from build123d import *

# Parameters (mm, degrees)
F1_DEPTH = 50
F2_DEPTH = 25
F0_W     = 36
F0_H     = 20
F3_DEPTH = 10
F4_DEPTH = 10


with BuildPart() as f1:
    # F0 (on Front) → F1 (new body, symmetric)
    with BuildSketch(Plane.XZ):
        Polygon((-60, -30), (60, -30), (60, 30), (18, 30), (18, 10), (-18, 10), (-18, 30), (-60, 30), align=None)
    extrude(amount=F1_DEPTH, both=True)

    # F0 (on Front) → F2 (join, symmetric)
    with BuildSketch(Plane.XZ):
        with BuildLine():
            add(Edge.make_bspline(
                [(-60, 30), (-60, 40.4474846921), (-37.2177352662, 50), (-18, 50)],
                knots=[0, 0, 0, 0, 46.5188133985, 46.5188133985, 46.5188133985, 46.5188133985], degree=3))
            Line((-60, 30), (-18, 30))
            Line((-18, 30), (-18, 50))
        make_face()
    extrude(amount=F2_DEPTH, both=True)

    # F0 (on Front) → F3 (join, symmetric)
    with BuildSketch(Plane.XZ):
        with Locations((0, 20)):
            Rectangle(F0_W, F0_H)
    extrude(amount=F3_DEPTH, both=True)

    # F0 (on Front) → F4 (join, symmetric)
    with BuildSketch(Plane.XZ):
        with Locations((0, 40)):
            Rectangle(F0_W, F0_H)
        with BuildLine():
            Line((18, 30), (60, 30))
            Line((60, 30), (60, 56.5))
            ThreePointArc((60, 56.5), (63.954058454, 66.045941546), (73.5, 70))
            Line((73.5, 70), (87.8666490715, 70))
            Line((87.8666490715, 70), (87.8666490715, 75))
            add(Edge.make_bspline(
                [(18, 50), (18.3067479085, 75.1533858136), (72.5292141174, 78.3742428055), (87.8666490715, 75)],
                knots=[0, 0, 0, 0, 74.2047751326, 74.2047751326, 74.2047751326, 74.2047751326], degree=3))
            Line((18, 50), (18, 30))
        make_face()
    extrude(amount=F4_DEPTH, both=True)

    # F0 (on Front) → F5 (revolve)
    with BuildSketch(Plane.XZ):
        Polygon((97.8666490715, 75), (87.8666490715, 75), (87.8666490715, 70), (92.8666490715, 70), (92.8666490715, 65), (97.8666490715, 65), align=None)
    revolve(axis=Axis((87.8666490715, 0, 70), (0, 0, 1)))


solid = f1.part
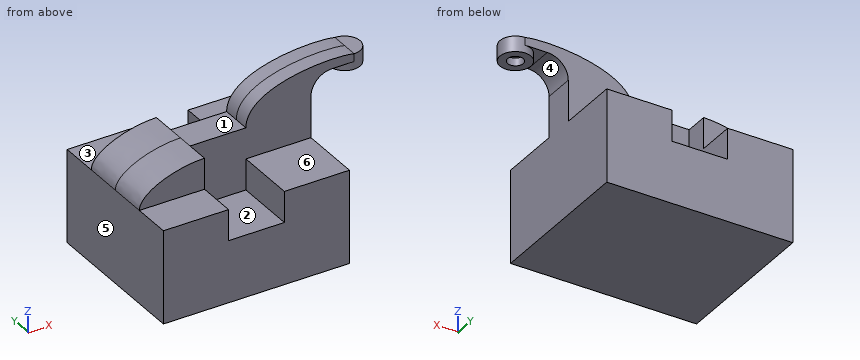
Input: part model. Units: mm. Frame: model coordinates. Face numbers are marked on the shaded views. A direction names the side the tool comes from. Coordinates: 2 decimals unless noted, no trailing zeros. Loops run counter-clockwise (first coordinate to the right, second up) from the corner with the lowest first, then second, coordinate; pieces in that order, holes last. Notation, with made-up numbers: (6, 23.5) -> (59, 23.5) arc R24 cw to (59, 62.5) -> close; hole circle Ø5 at (34, 2). An arc over 180 degrees is marked (long way). Write item = value, one per line. Start each with the question number.
Item 1: Reachability of the marked faces 1, 2 and 3 from +Z, -Z, +X, -X, +Y, -Y: full face, straight path, thin tool, end or side. Return the list, or none.
Item 2: Mould query, pull axis X, two halves, no side actions, for the marked faces 4, 5 and 6. Classes: pulls with the +X half, pulls with the -X half, needs draft (parallel to the pull), parting line crosses it, or undercut.
Item 3: Cut plane A-A, the plane z = 21. Return loops of the section in (x, y), plus the area to 3 significant figures.
Item 4: First-contact query: P1, Ø13, axis at x = 87.87, y = 0, coming from the +Z side; P2, Ø5, axis at y = 2, z = 54.5, coming from the +X side; P3, Ø11, axis at x = 88.5, y = 0.5, coming from the -Z side. Flat tips, straight axial feed; report the tip coordinate or a pass-through.
Item 5: Material intervals for line 1 (X direction, y = 42, z = 28.5); line 2 (Z direction, x = 16, y = -6); line 3 (X direction, y = -12, z = -18), sorted ascending.
Item 6: Cut plane B-B, the plane z = -18. Return loops of the section in (x, y).
Ans:
q1.face_1 = +Z, -X, +Y, -Y
q1.face_2 = +Z, -Y
q1.face_3 = +Z, +X, -X, +Y
q2.face_4 = undercut
q2.face_5 = pulls with the -X half
q2.face_6 = needs draft
q3.outline = (-60, -50) -> (-18, -50) -> (-18, -10) -> (18, -10) -> (18, -50) -> (60, -50) -> (60, 50) -> (18, 50) -> (18, 10) -> (-18, 10) -> (-18, 50) -> (-60, 50) -> close
q3.area = 9,120 mm²
q4.P1 = 75.86
q4.P2 = 60.01
q4.P3 = 65
q5.line_1 = -60 to -18, 18 to 60
q5.line_2 = -30 to 50
q5.line_3 = -60 to 60
q6.outline = (-60, -50) -> (60, -50) -> (60, 50) -> (-60, 50) -> close
